```python
from build123d import *

# Parameters (mm, degrees)
F0_W      = 2432.05
F0_H      = 387.35
F1_DEPTH  = 177.8
F6_W      = 76.2
F6_H      = 152.4
F7_DEPTH  = 34.925
F2_W      = 76.2
F2_H      = 152.4
F3_DEPTH  = 34.925
F8_DEPTH  = 422.275
F9_DEPTH  = 422.275
F4_W      = 76.2
F4_H      = 152.4
F10_DEPTH = 34.925
F5_DEPTH  = 422.275


with BuildPart() as f1:
    # F0 (on Top) → F1 (new body)
    with BuildSketch(Plane.XY):
        with Locations((770.752065, -1.466483)):
            Rectangle(F0_W, F0_H)
    extrude(amount=F1_DEPTH)

    # F6 (on face) → F7 (join)
    with BuildSketch(Plane.XZ.offset(195.141483)):
        with Locations((-292.872935, 88.9)):
            Rectangle(F6_W, F6_H)
    extrude(amount=F7_DEPTH)

    # F2 (on face) → F3 (join)
    with BuildSketch(Plane.XZ.offset(195.141483)):
        with Locations((1834.377065, 88.9)):
            Rectangle(F2_W, F2_H)
    extrude(amount=F3_DEPTH)

    # F2 (on face) → F8 (join)
    with BuildSketch(Plane.XZ.offset(195.141483)):
        with Locations((1834.377065, 88.9)):
            Rectangle(F2_W, F2_H)
    extrude(amount=-F8_DEPTH)

    # F6 (on face) → F9 (join)
    with BuildSketch(Plane.XZ.offset(195.141483)):
        with Locations((-292.872935, 88.9)):
            Rectangle(F6_W, F6_H)
    extrude(amount=-F9_DEPTH)

    # F4 (on face) → F10 (join)
    with BuildSketch(Plane.XZ.offset(195.141483)):
        with Locations((770.752065, 88.9)):
            Rectangle(F4_W, F4_H)
    extrude(amount=F10_DEPTH)

    # F4 (on face) → F5 (join)
    with BuildSketch(Plane.XZ.offset(195.141483)):
        with Locations((770.752065, 88.9)):
            Rectangle(F4_W, F4_H)
    extrude(amount=-F5_DEPTH)


solid = f1.part
```
Design review of the part built by this model. Coordinates are the model's own, in mm. Give positions to 0.01 mm unless a question says otherwise; leave off trailing zeros. Loops run counter-clockwise (first coordinate to the right, second up) from the corner with the lowest first, then second, coordinate; pieces in that order, holes last. Notation, with made-up numbers: M 83,-29.75 L 104,-29.75 A25 cw 104,-15.75 Z; hole C 41.25,33 d6. An arc over 180 degrees is marked long. Return JSON: item names as keys, results as strings. Group by question number.
Item 1: We need section A-A (z = 104.5). Give the boundary of the cut face in (x, y), and give its area (3 significant figures).
Item 2: Insertion check: pin 1 Ø10.5 at (x, y) = (-296.5, 217) entering from +Z; pin 2 Ø10.5 at (x, y) = (1818.5, -219) entering from -Z; pin 3 Ø6 at (x, z) = (1232, 56) entering from -Y; pin 4 Ø10 at (x, y) = (1374, -137.5) entering from -Z. Each pin has a flat end and moves straight along its axis. Give the tip position at first contact, or say it passes through.
Item 3: For probe 1 along X at (y, z) = (-196.5, 27); probe 2 along Y at (x, z) = (402, 116), list the stretches that pass through material, from the lowest coordinate up.
Item 4: We need section B-B (x = 17). Give the boundary of the cut face in (y, z), and give its area (3 significant figures).
Output:
{
 "1": {"outline": "M -445.27,-195.14 L -330.97,-195.14 L -330.97,-230.07 L -254.77,-230.07 L -254.77,-195.14 L 732.65,-195.14 L 732.65,-230.07 L 808.85,-230.07 L 808.85,-195.14 L 1796.28,-195.14 L 1796.28,-230.07 L 1872.48,-230.07 L 1872.48,-195.14 L 1986.78,-195.14 L 1986.78,192.21 L 1872.48,192.21 L 1872.48,227.13 L 1796.28,227.13 L 1796.28,192.21 L 808.85,192.21 L 808.85,227.13 L 732.65,227.13 L 732.65,192.21 L -254.77,192.21 L -254.77,227.13 L -330.97,227.13 L -330.97,192.21 L -445.27,192.21 Z", "area": "958,000 mm^2"},
 "2": {"pin 1": "stops at z = 165.1", "pin 2": "stops at z = 12.7", "pin 3": "stops at y = -195.14", "pin 4": "stops at z = 0"},
 "3": {"probe 1": "x = -330.97 to -254.77, 732.65 to 808.85, 1796.28 to 1872.48", "probe 2": "y = -195.14 to 192.21"},
 "4": {"outline": "M -195.14,0 L 192.21,0 L 192.21,177.8 L -195.14,177.8 Z", "area": "68,900 mm^2"}
}
